from build123d import *

# Parameters (mm, degrees)
BOSS_EXTRUDE1_DEPTH      = 6
BOSS_EXTRUDE1_DEPTH_BACK = 6
SKETCH1_R                = 72
SKETCH1_R_2              = 61
SKETCH5_R                = 2
CUT_EXTRUDE3_DEPTH       = 103.528044944
SKETCH6_W                = 20
SKETCH6_H                = 3
SKETCH6_W_2              = 3
SKETCH6_H_2              = 20
CUT_EXTRUDE4_DEPTH       = 103.528044944
SKETCH12_R               = 2
CUT_EXTRUDE8_DEPTH       = 158.495079274
SKETCH13_W               = 20
SKETCH13_H               = 3
SKETCH13_W_2             = 3
SKETCH13_H_2             = 20
CUT_EXTRUDE9_DEPTH       = 102.54801821
SKETCH15_R               = 4
CUT_EXTRUDE10_DEPTH      = 227.8695061
SKETCH16_R               = 4
CUT_EXTRUDE11_DEPTH      = 227.869506244
SKETCH17_R               = 4
CUT_EXTRUDE12_DEPTH      = 227.869506244
SKETCH18_R               = 4
CUT_EXTRUDE13_DEPTH      = 227.869506244
SKETCH19_R               = 2
CUT_EXTRUDE14_DEPTH      = 158.495079412


with BuildPart() as part:
    # Sketch1 → Boss-Extrude1 (new, two sides: drawn at the far end of the back side and taken through both)
    with BuildSketch(Plane(origin=(0, 0, 0), x_dir=(1, 0, 0), z_dir=(0, 1, 0)).offset(-BOSS_EXTRUDE1_DEPTH_BACK)):
        with Locations(Location((0, 0, 0), (0, 0, 270))):
            Circle(SKETCH1_R)
        with Locations(Location((0, 0, 0), (0, 0, 270))):
            Circle(SKETCH1_R_2, mode=Mode.SUBTRACT)
    extrude(amount=BOSS_EXTRUDE1_DEPTH + BOSS_EXTRUDE1_DEPTH_BACK)

    # Sketch5 → Cut-Extrude3 (cut, through all)
    with BuildSketch(Plane(origin=(0, 6, 0), x_dir=(1, 0, 0), z_dir=(0, 1, 0))):
        with Locations(Location((47.284209037, 47.284209037, 0), (0, 0, 270))):
            Circle(SKETCH5_R)
        with Locations(Location((47.284209037, -46.760992861, 0), (0, 0, 270))):
            Circle(SKETCH5_R)
        with Locations(Location((-46.760992861, -46.760992861, 0), (0, 0, 270))):
            Circle(SKETCH5_R)
        with Locations(Location((-46.760992861, 47.284209037, 0), (0, 0, 270))):
            Circle(SKETCH5_R)
    extrude(amount=-CUT_EXTRUDE3_DEPTH, mode=Mode.SUBTRACT)

    # Sketch6 → Cut-Extrude4 (cut, through all)
    with BuildSketch(Plane(origin=(0, 6, 0), x_dir=(1, 0, 0), z_dir=(0, 1, 0))):
        with Locations((0, -70.5)):
            Rectangle(SKETCH6_W, SKETCH6_H)
        with Locations((0, 70.5)):
            Rectangle(SKETCH6_W, SKETCH6_H)
        with Locations((70.5, 0)):
            Rectangle(SKETCH6_W_2, SKETCH6_H_2)
        with Locations((-70.5, 0)):
            Rectangle(SKETCH6_W_2, SKETCH6_H_2)
    extrude(amount=-CUT_EXTRUDE4_DEPTH, mode=Mode.SUBTRACT)

    # Sketch12 → Cut-Extrude8 (cut, through all)
    with BuildSketch(Plane.XY.offset(69)):
        with Locations((4, 3)):
            Circle(SKETCH12_R)
        with Locations((-4, 3)):
            Circle(SKETCH12_R)
        with Locations((4, -3)):
            Circle(SKETCH12_R)
        with Locations((-4, -3)):
            Circle(SKETCH12_R)
    extrude(amount=-CUT_EXTRUDE8_DEPTH, mode=Mode.SUBTRACT)

    # Sketch13 → Cut-Extrude9 (cut, through all)
    with BuildSketch(Plane(origin=(0, 6, 0), x_dir=(1, 0, 0), z_dir=(0, 1, 0))):
        with Locations((0, -60.5)):
            Rectangle(SKETCH13_W, SKETCH13_H)
        with Locations((0, 60.5)):
            Rectangle(SKETCH13_W, SKETCH13_H)
        with Locations((-60.5, 0)):
            Rectangle(SKETCH13_W_2, SKETCH13_H_2)
        with Locations((60.5, 0)):
            Rectangle(SKETCH13_W_2, SKETCH13_H_2)
    extrude(amount=-CUT_EXTRUDE9_DEPTH, mode=Mode.SUBTRACT)

    # Sketch15 → Cut-Extrude10 (cut, through all)
    with BuildSketch(Plane(origin=(-49.779681973, 6, -120.17878335), x_dir=(-0.9238795325112865, 0, 0.3826834323650906), z_dir=(-0.3826834323650906, 0, -0.9238795325112865))):
        with Locations((0, -6)):
            Circle(SKETCH15_R)
    extrude(amount=-CUT_EXTRUDE10_DEPTH, mode=Mode.SUBTRACT)

    # Sketch16 → Cut-Extrude11 (cut, through all)
    with BuildSketch(Plane(origin=(-120.17878335, 6, -49.779681973), x_dir=(-0.3826834323650807, 0, 0.9238795325112905), z_dir=(-0.9238795325112905, 0, -0.3826834323650807))):
        with Locations((0, -6)):
            Circle(SKETCH16_R)
    extrude(amount=-CUT_EXTRUDE11_DEPTH, mode=Mode.SUBTRACT)

    # Sketch17 → Cut-Extrude12 (cut, through all)
    with BuildSketch(Plane(origin=(-120.17878335, 6, 49.779681973), x_dir=(0.3826834323650807, 0, 0.9238795325112905), z_dir=(-0.9238795325112905, 0, 0.3826834323650807))):
        with Locations((0, -6)):
            Circle(SKETCH17_R)
    extrude(amount=-CUT_EXTRUDE12_DEPTH, mode=Mode.SUBTRACT)

    # Sketch18 → Cut-Extrude13 (cut, through all)
    with BuildSketch(Plane(origin=(-49.779681973, 6, 120.17878335), x_dir=(0.9238795325112865, 0, 0.3826834323650906), z_dir=(-0.3826834323650906, 0, 0.9238795325112865))):
        with Locations((0, -6)):
            Circle(SKETCH18_R)
    extrude(amount=-CUT_EXTRUDE13_DEPTH, mode=Mode.SUBTRACT)

    # Sketch19 → Cut-Extrude14 (cut, through all)
    with BuildSketch(Plane(origin=(69, 0, 0), x_dir=(0, 0, -1), z_dir=(1, 0, 0))):
        with Locations((4, 3)):
            Circle(SKETCH19_R)
        with Locations((-4, 3)):
            Circle(SKETCH19_R)
        with Locations((4, -3)):
            Circle(SKETCH19_R)
        with Locations((-4, -3)):
            Circle(SKETCH19_R)
    extrude(amount=-CUT_EXTRUDE14_DEPTH, mode=Mode.SUBTRACT)


solid = part.part
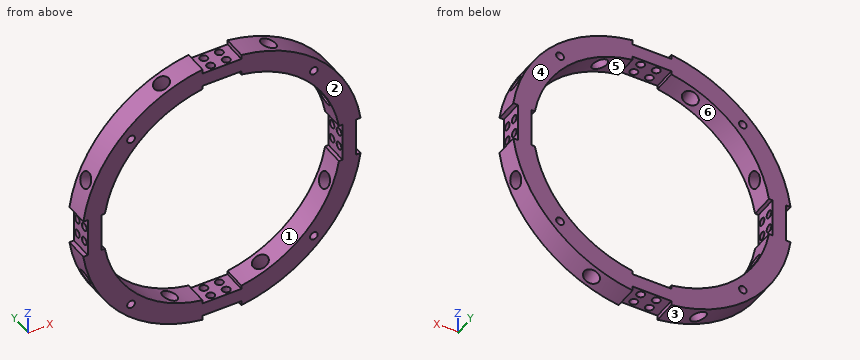
Design review of the part built by this model. Coordinates are the model's own, in mm. Face numbers are marked on the shaded views. A direction names the side the tool comes from. Coordinates: 2 decimals unless noted, no trailing zeros. Order: outer loops, then holes, each group sorted by start corner. A loop starts at its lowest first (then second) coordinate and runs counter-clockwise, first axis right, second up. Notation, with made-up numbers: (-28, -31) -> (-19, -31) arc R28 cw to (-19, -5) -> close; hole circle Ø10 at (-5.75, 58.25). An arc over 180 degrees is marked (long way). Use one line per item in the form item = value. Start each with the question number.
(1) Add section C-C on x = 42.5. State the section outline as (y, z) points, plus the area to 3 significant figures.
(2) Add section D-D on z = -41.5. State the section outline as (x, y) points, plus the area to 3 significant figures.
(3) Add section B-B on z = 4. State the section outline as (x, y) points.
(4) Insertion check: pin 1 (6.5 mm diameter, centred on y = -3, z = -4, fed in from +X); pin 2 (4 mm diameter, centred on x = 27, y = 3.5, fed in from +Z); pin 3 (2 mm diameter, centred on x = -61, y = 0, fed in from +Z). Each pin has a flat end and moves straight along its axis. Give the tip position at first contact, or say it passes through.
(5) For the marked faces 1 and 2, list the 3-axis set-ups (+Z, -Z, +X, -X, +Y, -Y) from which the entire face can be reached by the end or side of a thin tool; tool diameter is ignored.
(6) For probe 1 along Y at (x, z) = (4, 64.75); probe 2 along X at (y, z) = (4.5, -14); probe 3 along X at (y, z) = (3.5, -64.5), list the stretches that pass through material, from the lowest coordinate up.
(7) The part is to be moulded in two halves that separate along X. For the marked faces 3, 4, 5 and 6, say which applies: +X half, -X half, draft (parallel to the pull), parting line (faces both ways), or undercut.
(8) Add section A-A on x = -4. State the section outline as (y, z) points, plus the area to 3 significant figures.
Answer block:
q1.outline = (-6, -58.12) -> (6, -58.12) -> (6, -43.76) -> (-6, -43.76) -> close; (-6, 43.76) -> (6, 43.76) -> (6, 58.12) -> (-6, 58.12) -> close
q1.area = 345 mm²
q2.outline = (-58.84, -6) -> (-44.71, -6) -> (-44.71, 6) -> (-58.84, 6) -> close; (44.71, -6) -> (58.84, -6) -> (58.84, 6) -> (44.71, 6) -> close
q2.area = 339 mm²
q3.outline = (-69, -6) -> (-62, -6) -> (-62, -5) -> (-69, -5) -> close; (-69, -1) -> (-62, -1) -> (-62, 1) -> (-69, 1) -> close; (-69, 5) -> (-62, 5) -> (-62, 6) -> (-69, 6) -> close; (62, -6) -> (69, -6) -> (69, -5) -> (62, -5) -> close; (62, -1) -> (69, -1) -> (69, 1) -> (62, 1) -> close; (62, 5) -> (69, 5) -> (69, 6) -> (62, 6) -> close
q4.pin_1 = 69
q4.pin_2 = 67.52
q4.pin_3 = 39.8
q5.face_1 = +Y, -Y
q5.face_2 = +Z, -Z, +X, -X, -Y
q6.probe_1 = -6 to -5, -1 to 1, 5 to 6
q6.probe_2 = -70.63 to -59.37, 59.37 to 70.63
q6.probe_3 = -32 to -28.81, -24.62 to -5.94, -2.06 to 2.06, 5.94 to 24.62, 28.81 to 32
q7.face_3 = -X half
q7.face_4 = draft
q7.face_5 = undercut
q7.face_6 = undercut
q8.outline = (-6, -69) -> (-5, -69) -> (-5, -62) -> (-6, -62) -> close; (-6, 62) -> (-5, 62) -> (-5, 69) -> (-6, 69) -> close; (-1, -69) -> (1, -69) -> (1, -62) -> (-1, -62) -> close; (-1, 62) -> (1, 62) -> (1, 69) -> (-1, 69) -> close; (5, -69) -> (6, -69) -> (6, -62) -> (5, -62) -> close; (5, 62) -> (6, 62) -> (6, 69) -> (5, 69) -> close
q8.area = 56.0 mm²
